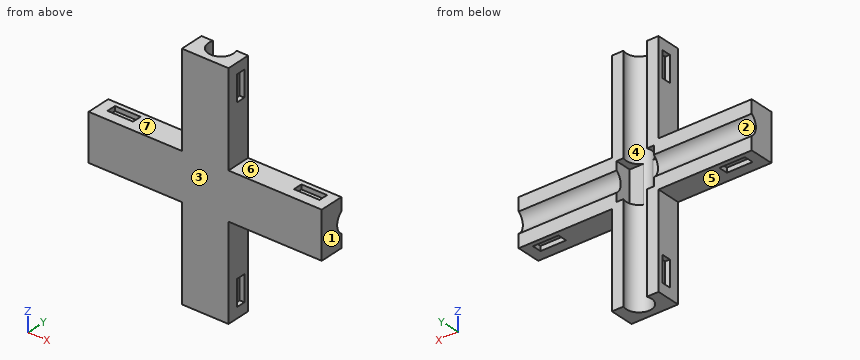
from build123d import *

# Parameters (mm, degrees)
BOSS_EXTRUDE5_DEPTH         = 5.2
CUT_EXTRUDE1_REACH          = 58.143
SKETCH4_R                   = 2.7
SKETCH5_R                   = 2.7
CUT_EXTRUDE2_DEPTH          = 57.143031625
SKETCH6_W                   = 8
SKETCH6_H                   = 8
CUT_EXTRUDE3_DEPTH          = 3.5
SKETCH7_W                   = 5.5
SKETCH7_H                   = 2
CUT_EXTRUDE4_DEPTH          = 1
CIRPATTERN1_COUNT           = 4
CIRPATTERN1_COPY_1_SKETCH_W = 5.5
CIRPATTERN1_COPY_1_SKETCH_H = 2
CIRPATTERN1_COPY_1_DEPTH    = 1
CIRPATTERN1_COPY_2_SKETCH_W = 5.5
CIRPATTERN1_COPY_2_SKETCH_H = 2
CIRPATTERN1_COPY_2_DEPTH    = 1
CIRPATTERN1_COPY_3_SKETCH_W = 5.5
CIRPATTERN1_COPY_3_SKETCH_H = 2
CIRPATTERN1_COPY_3_DEPTH    = 1


with BuildPart() as part:
    # Sketch3 → Boss-Extrude5 (new body)
    with BuildSketch(Plane(origin=(0, 0, 0), x_dir=(1, 0, 0), z_dir=(0, 1, 0))):
        Polygon((5, 5), (25, 5), (25, -5), (5, -5), (5, -25), (-5, -25), (-5, -5), (-25, -5), (-25, 5), (-5, 5), (-5, 25), (5, 25), align=None)
    extrude(amount=BOSS_EXTRUDE5_DEPTH)

    # Sketch4 → Cut-Extrude1 (cut, up to next)
    with BuildSketch(Plane.XY.offset(25), mode=Mode.PRIVATE) as cut_extrude1_sk1:
        with Locations((0, 4.2)):
            Circle(SKETCH4_R)
    cut_extrude1_tool1 = extrude(cut_extrude1_sk1.sketch, amount=-CUT_EXTRUDE1_REACH, mode=Mode.PRIVATE) & part.part
    add(cut_extrude1_tool1.solids().sort_by_distance((0, 4.2, 25))[0], mode=Mode.SUBTRACT)

    # Sketch5 → Cut-Extrude2 (cut, through all)
    with BuildSketch(Plane(origin=(25, 0, 0), x_dir=(0, 0, -1), z_dir=(1, 0, 0))):
        with Locations((0, 6.8)):
            Circle(SKETCH5_R)
    extrude(amount=-CUT_EXTRUDE2_DEPTH, mode=Mode.SUBTRACT)

    # Sketch6 → Cut-Extrude3 (cut)
    with BuildSketch(Plane(origin=(0, 5.2, 0), x_dir=(1, 0, 0), z_dir=(0, 1, 0))):
        Rectangle(SKETCH6_W, SKETCH6_H)
    extrude(amount=-CUT_EXTRUDE3_DEPTH, mode=Mode.SUBTRACT)

    # Sketch7 → Cut-Extrude4 (cut)
    with BuildSketch(Plane.XY.offset(5)):
        with Locations((20, 3.2)):
            Rectangle(SKETCH7_W, SKETCH7_H)
    cut_extrude4 = extrude(amount=-CUT_EXTRUDE4_DEPTH, mode=Mode.SUBTRACT)

    # Mirror1: Cut-Extrude4 across plane
    add(cut_extrude4.mirror(Plane.XY), mode=Mode.SUBTRACT)

    # CirPattern1: Cut-Extrude4 ×4 about axis
    cirpattern1_axis = Axis((0, 0, 0), (0, 1, 0))
    for i in range(1, CIRPATTERN1_COUNT):
        add(cut_extrude4.rotate(cirpattern1_axis, i * 360 / CIRPATTERN1_COUNT), mode=Mode.SUBTRACT)

    # CirPattern1 copy 1 sketch → CirPattern1 copy 1 (cut)
    with BuildSketch(Plane(origin=(-5, 0, 0), x_dir=(0, 0, -1), z_dir=(-1, 0, 0))):
        with Locations((20, -3.2)):
            Rectangle(CIRPATTERN1_COPY_1_SKETCH_W, CIRPATTERN1_COPY_1_SKETCH_H)
    extrude(amount=-CIRPATTERN1_COPY_1_DEPTH, mode=Mode.SUBTRACT)

    # CirPattern1 copy 2 sketch → CirPattern1 copy 2 (cut)
    with BuildSketch(Plane(origin=(0, 0, 5), x_dir=(-1, 0, 0), z_dir=(0, 0, 1))):
        with Locations((20, -3.2)):
            Rectangle(CIRPATTERN1_COPY_2_SKETCH_W, CIRPATTERN1_COPY_2_SKETCH_H)
    extrude(amount=-CIRPATTERN1_COPY_2_DEPTH, mode=Mode.SUBTRACT)

    # CirPattern1 copy 3 sketch → CirPattern1 copy 3 (cut)
    with BuildSketch(Plane(origin=(5, 0, 0), x_dir=(0, 0, 1), z_dir=(1, 0, 0))):
        with Locations((20, -3.2)):
            Rectangle(CIRPATTERN1_COPY_3_SKETCH_W, CIRPATTERN1_COPY_3_SKETCH_H)
    extrude(amount=-CIRPATTERN1_COPY_3_DEPTH, mode=Mode.SUBTRACT)


solid = part.part
The model under review builds one solid part; all positions refer to its coordinate system, in mm. Face numbers are marked on the shaded views. A direction names the side the tool comes from. Round coordinates to 2 decimals unless told otherwise and drop trailing zeros. Loops run counter-clockwise (first coordinate to the right, second up) from the corner with the lowest first, then second, coordinate; pieces in that order, holes last. Notation, with made-up numbers: (-4, -37.75) -> (4, -37.75) arc R18 ccw to (4, -18.75) -> close; hole circle Ø2 at (-21.75, -13.5). An arc over 180 degrees is marked (long way). One line per question, with ' | ' between items. Start each with the question number.
Item 1: Add section D-D, the plane x = -14. Write out the cut boundary in (y, z), then the cut area to 3 significant figures.
Item 2: Add section C-C, the plane z = 7. Write out the cut boundary in (x, y).
Item 3: Machinability: for the marked faces 5, 6 and 7, which of the approach directions +Z, -Z, +X, -X, +Y, -Y give a long, thin tool a straight path to every point of the face, cutting with its end or side? Answer none if there is none.
Item 4: Draft analysis for pull direction Y (two halves, no side actions). For the marked faces 1, 2, 3 and 4, state which applies: +Y half, -Y half, draft (parallel to the pull), parting line (faces both ways), or undercut.
Item 5: Wall thickness on line 1 along X through (y, z) = (4.2, -2.5); line 2 along X through (y, z) = (4.2, -7); line 3 along Y through (x, z) = (0, -8): over which ranges is each line inside the solid? List them lowest first. Write a range as [from, to].
Item 6: Add section B-B, the plane y = 0.8. Write out the cut boundary in (x, z).
Item 7: Add section A-A, the plane x = 20. Write out the cut boundary in (y, z).
Item 8: For pin 1 (0.6 mm diameter, centred on y = 3, z = -21, fed in from -X); pin 2 (1 mm diameter, centred on y = 4, z = 17, fed in from -X); pin 3 (1 mm diameter, centred on x = 21, y = 3, fed in from +Z), all flat-tipped, find the tip position at first contact; note any pin that passes through.
Return value:
1) outline: (0, -5) -> (5.2, -5) -> (5.2, -2.17) arc R2.7 cw to (5.2, 2.17) -> (5.2, 5) -> (0, 5) -> close | area: 48.7 mm2
2) outline: (-5, 0) -> (5, 0) -> (5, 5.2) -> (2.51, 5.2) arc R2.7 cw (long way) to (-2.51, 5.2) -> (-5, 5.2) -> close
3) face 5: -Z, -X, +Y, -Y | face 6: +Z, +X, +Y, -Y | face 7: +Z, -X, +Y, -Y
4) face 1: draft | face 2: +Y half | face 3: -Y half | face 4: undercut
5) line 1: x = [-25, -4], [4, 25] | line 2: x = [-5, -2.7], [2.7, 5] | line 3: y = [0, 1.5]
6) outline: (-25, -5) -> (-5, -5) -> (-5, -25) -> (5, -25) -> (5, -5) -> (25, -5) -> (25, 5) -> (5, 5) -> (5, 25) -> (-5, 25) -> (-5, 5) -> (-25, 5) -> close
7) outline: (0, -5) -> (2.2, -5) -> (2.2, -4) -> (4.2, -4) -> (4.2, -5) -> (5.2, -5) -> (5.2, -2.17) arc R2.7 cw to (5.2, 2.17) -> (5.2, 5) -> (4.2, 5) -> (4.2, 4) -> (2.2, 4) -> (2.2, 5) -> (0, 5) -> close
8) pin 1: stops at x = -4 | pin 2: stops at x = -5 | pin 3: stops at z = 4
